Solid Edge part; units mm, degrees
sketch "Sketch1" plane through (0, 0, 0) normal (1, 0, 0) x (0, 1, 0)
  line L0 (7.5, 30) -> (-7.5, 30)
  line L1 (-7.5, 30) -> (-7.5, -30)
  line L2 (-7.5, -30) -> (7.5, -30)
  line L3 (7.5, -30) -> (7.5, 30)
extrude "largo" add sketch "Sketch1" along normal mid plane 132
hole "Hole1" at (30.5, 7.5, 15) direction (0, -1, 0) diameter 8 end up to next
hole "Hole2" at (-30.5, 7.5, 15) direction (0, -1, 0) diameter 8 end up to next
sketch "Sketch2" plane through (66, 0, 0) normal (1, 0, 0) x (0, 1, 0)
  arc A0 (-48.5, -11) -> (-32.7514, -10.5193) centre (-40.1119, -27.5899) cw
  line L0 (-48.5, -20) -> (-48.5, -11)
  line L1 (-7.5, -20) -> (-48.5, -20)
  line L2 (-7.5, 21) -> (-7.5, -20)
  line L3 (-48.5, 21) -> (-7.5, 21)
  line L4 (-48.5, 21) -> (-48.5, 12)
  arc A1 (-48.5, 12) -> (-32.7514, 11.5193) centre (-40.1119, 28.5899) ccw
  arc A2 (-32.7514, 11.5193) -> (-32.7514, -10.5193) centre (-28, 0.5) cw
extrude "Protrusion1" add sketch "Sketch2" against normal blind 6
hole "Agujero_7" at (60, -12.5, 16) direction (1, 0, 0) diameter 6 end up to next
hole "Hole3" at (60, -43.5, 16) direction (1, 0, 0) diameter 6 end up to next
hole "Hole4" at (60, -43.5, -15) direction (1, 0, 0) diameter 6 end up to next
hole "Hole5" at (60, -12.5, -15) direction (1, 0, 0) diameter 6 end up to next
fillet "Redondeo_1" radius 2 7 edges at (0, 7.5, 30) (0, -7.5, 30) (-66, 7.5, 0) (-66, -7.5, 0) (66, 7.5, 0) (66, 0, 30) (-66, 0, 30)
Work out the finished part from the listing and answer in its coordinate system (mm). A direction names the side the tool comes from. Give positions to 0.01 mm unless a question says otherwise; leave off trailing zeros. Loops run counter-clockwise (first coordinate to the right, second up) from the corner with the lowest first, then second, coordinate; pieces in that order, holes last. Notation, with made-up numbers: (77.5, 16) -> (98.5, 16) arc R17 cw to (98.5, 22) -> close; hole circle Ø8 at (38.5, 45). An arc over 180 degrees is marked (long way). Use a Markdown table: item, result. Add a question column.
1. Find the intervals of material crossed by probe 1 along X at (y, z) = (-3, 15); probe 2 along Y at (x, z) = (61, 16); probe 3 along Z at (x, y) = (64.6, -12.5), in increasing order.
2. Section D-D on z = 24 is taken. Determine the outline of the cut face in (x, y).
3. Flat-ended cylindrical pins translate along their axes: pin 1 Ø12 at (x, z) = (5, 19.5) entering from -Y; pin 2 Ø6.5 at (x, y) = (64, -33) entering from +Z; pin 3 Ø7 at (y, z) = (-12.5, 16) entering from -X. Find the tip coordinate at first contact, or state that the pin passes through.
4. Section C-C on z = 15 is taken. Determine the outline of the cut face in (x, y), and give its area (3 significant figures).
5. Section B-B on x = 30.5 is taken. Determine the outline of the cut face in (y, z), and give its area (3 significant figures).
6. For faces 4 (the flat face through (63, -28, -20)), 5 (the flat face through (-1, 0, 30)), 6 (the cylindrical face through (63.042, -40.565, -9.005)), determine the directions among +Z, -Z, +X, -X, +Y, -Y from which every point of the face is accessible in a straight line to the end or side of a thin tool.
7. Section A-A on y = -12.5 is taken. Determine the outline of the cut face in (x, z).
8. Determine the mould class of faces 1 (the flat face through (60, -15, 1)), 2 (the flat face through (63, -28, 21)), 3 (the cylindrical face through (34.466, 0.105, 14.479)) for opening direction Z: released by +Z, released by -Z, zero draft, split by the parting line, or undercut.
Results below:
| question | item | result |
|---|---|---|
| 1 | probe 1 | x = -66 to -34.5, -26.5 to 26.5, 34.5 to 66 |
| 1 | probe 2 | y = -48.5 to -46.5, -40.5 to -15.5, -9.5 to 7.5 |
| 1 | probe 3 | z = -20 to -18, -12 to 13, 19 to 21 |
| 2 | outline | (-66, -5.5) arc R2 ccw to (-64, -7.5) -> (66, -7.5) -> (66, 5.5) arc R2 ccw to (64, 7.5) -> (-64, 7.5) arc R2 ccw to (-66, 5.5) -> close |
| 3 | pin 1 | stops at y = -7.5 |
| 3 | pin 2 | stops at z = 21 |
| 3 | pin 3 | stops at x = 60 |
| 4 | outline | (-66, -5.5) arc R2 ccw to (-64, -7.5) -> (-34.5, -7.5) -> (-34.5, 7.5) -> (-64, 7.5) arc R2 ccw to (-66, 5.5) -> close; (-26.5, -7.5) -> (26.5, -7.5) -> (26.5, 7.5) -> (-26.5, 7.5) -> close; (34.5, -7.5) -> (60, -7.5) -> (60, -9.67) -> (66, -9.67) -> (66, 5.5) arc R2 ccw to (64, 7.5) -> (34.5, 7.5) -> close; (60, -48.5) -> (66, -48.5) -> (66, -46.33) -> (60, -46.33) -> close; (60, -40.67) -> (66, -40.67) -> (66, -15.33) -> (60, -15.33) -> close |
| 4 | area | 1,920 mm^2 |
| 5 | outline | (-7.5, -30) -> (7.5, -30) -> (7.5, 11) -> (-7.5, 11) -> close; (-7.5, 19) -> (7.5, 19) -> (7.5, 28) arc R2 ccw to (5.5, 30) -> (-5.5, 30) arc R2 ccw to (-7.5, 28) -> close |
| 5 | area | 778 mm^2 |
| 6 | face 4 | -Z, +X, -X, -Y |
| 6 | face 5 | +Z, +X, -X, +Y, -Y |
| 6 | face 6 | +X, -X |
| 7 | outline | (60, -20) -> (66, -20) -> (66, -18) -> (60, -18) -> close; (60, -12) -> (66, -12) -> (66, 13) -> (60, 13) -> close; (60, 19) -> (66, 19) -> (66, 21) -> (60, 21) -> close |
| 8 | face 1 | zero draft |
| 8 | face 2 | released by +Z |
| 8 | face 3 | undercut |
